Autodesk Inventor part; units mm, degrees
ref_plane "YZ Plane" through (0, 0, 0) normal (1, 0, 0) x (0, 1, 0)
ref_plane "XZ Plane" through (0, 0, 0) normal (0, 1, 0) x (-1, 0, 0)
ref_plane "XY Plane" through (0, 0, 0) normal (0, 0, 1) x (1, 0, 0)
sketch "Sketch1" plane through (0, 0, 0) normal (0, 0, 1) x (1, 0, 0)
  line L0 (-28.59, -15) -> (28.59, -15)
  line L1 (28.59, -15) -> (28.59, 15)
  line L2 (28.59, 15) -> (-28.59, 15)
  line L3 (-28.59, 15) -> (-28.59, -15)
  line L4 (-28.59, -15) -> (28.59, 15) construction
  line L5 (28.59, -15) -> (-28.59, 15) construction
  point P0 (0, 0)
  dimension "d0" = 57.18
  dimension "d1" = 30
extrude "Plate1" add sketch "Sketch1" along normal blind 1.5
sketch "Sketch2" plane through (-27.09, -15, 0) normal (-1, 0, 0) x (0, -1, 0)
  line L0 (-30, 0) -> (0, 0)
  line L1 (0, 0) -> (0, 45)
  line L2 (0, 45) -> (-30, 45)
  line L3 (-30, 45) -> (-30, 0)
edge flange "Flange1" height 45 angle 90 thickness 1.5 bend radius 0.31 thickness toward (-1, 0, 0) relief tear relief width 1.5 relief depth 0.75 corner gap 0.31 corner form 0 edges at (-28.59, 0, 1.5) (28.59, 0, 1.5) wall of the first edge with corners at (-27.09, 15, 0) (-27.09, -15, 0) (-27.09, -15, 45) (-27.09, 15, 45)
bend "Bend1"
corner "Corner1"
sketch "Sketch3" plane through (28.59, -15, 45) normal (1, 0, 0) x (0, 0, -1)
  circle A0 centre (17, 15) radius 9.96
  line L0 (0, 30) -> (43.19, 30)
  line L1 (43.19, 0) -> (0, 0)
  line L2 (31.19, 30) -> (13.9636, 24.4859)
  line L3 (31.19, 0) -> (13.9636, 5.5141)
  line L4 (0, 30) -> (0, 0)
  point P0 (45, 15)
  dimension "d13" = 19.92
  dimension "d14" = 12
  dimension "d15" = 28
extrude "Cut1" cut sketch "Sketch3" against normal blind 57.18 contours A0 L3 L1 L4 L0 L2
equation "\"d2\" = Thickness"
equation "\"d3\" = BendReliefWidth"
equation "\"d4\" = BendReliefDepth"
equation "\"d5\" = MinimumRemnant"
equation "\"d6\" = TransitionRadius"
equation "\"d9\" = BendRadius"
equation "\"d10\" = CornerReliefSize"
equation "\"d11\" = GapSize"
equation "\"d12\" = JacobiRadiusSize"
equation "\"BendReliefWidth\" = Thickness"
equation "\"BendReliefDepth\" = 0.5 * Thickness"
equation "\"CornerReliefSize\" = 4 * Thickness"
equation "\"MinimumRemnant\" = 2 * Thickness"
equation "\"TransitionRadius\" = BendRadius"
equation "\"JacobiRadiusSize\" = BendRadius"
equation "\"GapSize\" = Thickness"
properties part number "axis_21_bottom_frame" material "Aluminum 6061-AHC"
Part model, mm, in its own coordinate system. A direction names the side the tool comes from. Give positions to 0.01 mm unless a question says otherwise; leave off trailing zeros. Order: outer loops, then holes, each group sorted by start corner. A loop starts at its lowest first (then second) coordinate and runs counter-clockwise, first axis right, second up. Notation, with made-up numbers: M -30,12.5 L -21,12.5 A18 cw -21,33.5 Z; hole C -17,15.5 d6. An arc over 180 degrees is marked long. Use a Markdown table: item, result. Add a question column.
(1) 3-axis set-ups, long thin cutter, end or side, ignore diameter. For faces 4 (the face through (-27.09, 0, 16)), 5 (the face through (-27.83, -12.282, 22.303)): which of +Z, -Z, +X, -X, +Y, -Y reach the whole face in a straight line?
(2) Saw through at B-B, the plane y = -7. Give the cut face in (x, z).
(3) Saw through at A-A, the plane z = 7. Give the cut face in (x, y).
(4) Probe line 1 along X through (y, z) = (-6, 26.5); line 2 along Z through (x, y) = (9.5, 0). List the from-to ranges inside material, lowest first. Write a range as [from, to].
(5) Drop flat-ended pins along their axis: P1, Ø5, axis at x = -11, y = 5.5, coming from the +Z side; P2, Ø6, axis at x = 8, y = -3.5, coming from the -Z side. Give the stop position or say it passes through.
(6) Saw through at C-C, the plane z = 14.5. Give the cut face in (x, y), and give its area (3 significant figures).
(7) Mould opens along X. For faces 1 (the face through (0, 15, 1)), 2 (the face through (0, 0, 1.5)), 3 (the face through (-28.07, -0.21, 0.54)) say: +X half, -X half, draft (parallel to the pull), parting line (faces both ways), or undercut.
(8) Saw through at D-D, the plane x = -17. Give the cut face in (y, z).
Answer key:
| question | item | result |
|---|---|---|
| 1 | face 4 | +Z, +Y, -Y |
| 1 | face 5 | +Z, +X, -X, -Y |
| 2 | outline | M -28.59,1.81 A1.81 ccw -26.78,0 L 26.78,0 A1.81 ccw 28.59,1.81 L 28.59,35.09 L 27.09,35.09 L 27.09,1.81 A0.31 cw 26.78,1.5 L -26.78,1.5 A0.31 cw -27.09,1.81 L -27.09,35.09 L -28.59,35.09 Z |
| 3 | outline | M -28.59,-15 L -27.09,-15 L -27.09,15 L -28.59,15 Z; M 27.09,-15 L 28.59,-15 L 28.59,15 L 27.09,15 Z |
| 4 | line 1 | [-28.59, -27.09], [27.09, 28.59] |
| 4 | line 2 | [0, 1.5] |
| 5 | P1 | z = 1.5 |
| 5 | P2 | z = 0 |
| 6 | outline | M -28.59,-14.78 L -27.09,-14.78 L -27.09,14.78 L -28.59,14.78 Z; M 27.09,-14.78 L 28.59,-14.78 L 28.59,14.78 L 27.09,14.78 Z |
| 6 | area | 88.7 mm^2 |
| 7 | face 1 | draft |
| 7 | face 2 | undercut |
| 7 | face 3 | -X half |
| 8 | outline | M -15,0 L 15,0 L 15,1.5 L -15,1.5 Z |
